```python
from build123d import *

# Parameters (mm, degrees)
SKETCH_1_R          = 1.5
EXTRUDE_1_DEPTH     = 3.8
SKETCH_2_OUTSIDE_W  = 9.992
SKETCH_2_OUTSIDE_H  = 9.736
SKETCH_2_OUTSIDE_R  = 2.219238474
CUT_EXTRUDE_1_DEPTH = 1
FILLET_1_R          = 0.3


with BuildPart() as part:
    # 草图1 → 凸台-拉伸1 (new body)
    with BuildSketch(Plane.XY):
        Polygon((-1.042677443, 2.938166733), (-3.065865753, 0.566098213), (-2.02318831, -2.37206852), (1.042677443, -2.938166733), (3.065865753, -0.566098213), (2.02318831, 2.37206852), align=None)
        with Locations(Location((0, 0, 0), (0, 0, 180))):
            Circle(SKETCH_1_R, mode=Mode.SUBTRACT)
    extrude(amount=EXTRUDE_1_DEPTH)

    # 草图2 outside → 切除-拉伸1 (cut)
    with BuildSketch(Plane(origin=(0, 0, 0), x_dir=(-1, 0, 0), z_dir=(0, 0, -1))):
        Rectangle(SKETCH_2_OUTSIDE_W, SKETCH_2_OUTSIDE_H)
        Circle(SKETCH_2_OUTSIDE_R, mode=Mode.SUBTRACT)
    extrude(amount=-CUT_EXTRUDE_1_DEPTH, mode=Mode.SUBTRACT)

    # 圆角1
    fillet_1_edges = [part.edges().sort_by_distance(p)[0] for p in [
        (2.219238474, 0, 0),
    ]]
    fillet(fillet_1_edges, radius=FILLET_1_R)


solid = part.part
```
The listing builds one solid part. Answer for the finished solid, in the listing's coordinates (mm). A direction names the side the tool comes from. Give positions to 0.01 mm unless a question says otherwise; leave off trailing zeros. Write each loop counter-clockwise with the first axis right and the second up, starting at its lowest first coordinate (ties: lowest second). Pieces come first, ordered by that corner, then holes. Notation, with made-up numbers: (10, 10) -> (65, 10) arc R20 ccw to (65, 41) -> close; hole circle Ø7 at (24, 28). An arc over 180 degrees is marked (long way). Write item = value, one per line. Start each with the question number.
1) The part is cut by section B-B, the plane x = 0. Determine the outline of the cut face in (y, z), and give its area (3 significant figures).
2) The part is cut by section A-A, the plane z = 1.3. Determine the outline of the cut face in (x, y).
3) The part is cut by section C-C, the plane y = 0. Determine the outline of the cut face in (x, z), and give its area (3 significant figures).
4) Straight lines are drawn through the part: line 1 along Z through (x, y) = (2, 1.3); line 2 along Y through (x, z) = (0, 1.25); line 3 along Y through (x, z) = (0.5, 0.65). For each, find the intervals that lie inside material, in ascending order.
5) Which of the six approach directions +Z, -Z, +X, -X, +Y, -Y give full straight-line access (tool end or side, diameter ignored) to faces 1 (the face through (-2.117, 0.667, 0.645)), 2 (the face through (-2.552, -0.882, 2.38))?
6) Each of these flat-tipped pins is pushed along its axis until it touches: pin 1 (1.8 mm diameter, centred on x = -0.5, y = -0.5, fed in from -Z); pin 2 (2.5 mm diameter, centred on x = 0, y = 0, fed in from -Z); pin 3 (2 mm diameter, centred on y = 2, z = 3, fed in from +X); pin 4 (1.5 mm diameter, centred on x = -2, z = 3, fed in from -Y). Where does it stop, or does it pass through?
7) Determine the mould class of faces 3 (the face through (0.51, 2.65, 2.38)), 4 (the face through (-2.04, 1.77, 2.38)), 5 (the face through (-1.43, -0.45, 1.87)) for opening direction X: +X half, -X half, draft (parallel to the pull), parting line (faces both ways), or undercut.
8) The part is cut by section D-D, the plane z = 0.7. Determine the outline of the cut face in (x, y), and give its area (3 significant figures).
Solutions:
q1.outline = (-2.75, 1) -> (-2.22, 1) -> (-2.22, 0.3) arc R0.3 ccw to (-1.92, 0) -> (-1.5, 0) -> (-1.5, 3.8) -> (-2.75, 3.8) -> close; (1.5, 0) -> (1.92, 0) arc R0.3 ccw to (2.22, 0.3) -> (2.22, 1) -> (2.75, 1) -> (2.75, 3.8) -> (1.5, 3.8) -> close
q1.area = 8.38 mm²
q2.outline = (-3.07, 0.57) -> (-2.02, -2.37) -> (1.04, -2.94) -> (3.07, -0.57) -> (2.02, 2.37) -> (-1.04, 2.94) -> close; hole circle Ø3 at (0, 0)
q3.outline = (-2.86, 1) -> (-2.22, 1) -> (-2.22, 0.3) arc R0.3 ccw to (-1.92, 0) -> (-1.5, 0) -> (-1.5, 3.8) -> (-2.86, 3.8) -> close; (1.5, 0) -> (1.92, 0) arc R0.3 ccw to (2.22, 0.3) -> (2.22, 1) -> (2.86, 1) -> (2.86, 3.8) -> (1.5, 3.8) -> close
q3.area = 9.04 mm²
q4.line_1 = 1 to 3.8
q4.line_2 = -2.75 to -1.5, 1.5 to 2.75
q4.line_3 = -2.16 to -1.41, 1.41 to 2.16
q5.face_1 = -Z
q5.face_2 = +Z, -Z, -X, -Y
q6.pin_1 = 0
q6.pin_2 = through
q6.pin_3 = 2.51
q6.pin_4 = -2.51
q7.face_3 = +X half
q7.face_4 = -X half
q7.face_5 = undercut
q8.outline = circle Ø4.44 at (0, 0); hole circle Ø3 at (0, 0)
q8.area = 8.40 mm²
